Autodesk Inventor part; units mm, degrees
ref_plane "YZ Plane" through (0, 0, 0) normal (1, 0, 0) x (0, 1, 0)
ref_plane "XZ Plane" through (0, 0, 0) normal (0, 1, 0) x (-1, 0, 0)
ref_plane "XY Plane" through (0, 0, 0) normal (0, 0, 1) x (1, 0, 0)
sketch "Эскиз1" plane through (0, 0, 0) normal (0, 0, 1) x (1, 0, 0)
  line L0 (0, 0) -> (10.2, 0)
  line L1 (10.2, 0) -> (10.2, -6.1)
  line L2 (10.2, -6.1) -> (0, -6.1)
  line L3 (0, -6.1) -> (0, 0)
  line L4 (10.2, -6.1) -> (2.2, -6.1)
  line L5 (2.2, -6.1) -> (2.2, -7.1)
  line L6 (2.2, -7.1) -> (10.2, -7.1)
  line L7 (10.2, -7.1) -> (10.2, -6.1)
  dimension "d0" = 10.2
  dimension "d1" = 6.1
  dimension "d2" = 8
  dimension "d3" = 1
extrude "Выдавливание1" add sketch "Эскиз1" along normal blind 0.8
sketch "Эскиз2" plane through (0, 0, 0.8) normal (0, 0, 1) x (1, 0, 0)
  line L0 (2.2, -7.1) -> (10.2, -7.1)
  line L1 (10.2, -7.1) -> (10.2, -3.9)
  line L2 (10.2, -7.1) -> (10.2, 0)
  line L3 (10.2, -3.9) -> (5.1, -3.9)
  line L4 (0, 0) -> (0, -6.1)
  circle A0 centre (5.1, -3.9) radius 1.9
  dimension "d6" = 3.2
  dimension "d7" = 5.1
  dimension "d8" = 3.8
extrude "Выдавливание2" cut sketch "Эскиз2" against normal blind 0.8
properties part number "shayba kvadrat"
Could you check a few things on this model? Use its own coordinates, in mm. Round coordinates to 2 decimals unless told otherwise and drop trailing zeros. Order: outer loops, then holes, each group sorted by start corner. A loop starts at its lowest first (then second) coordinate and runs counter-clockwise, first axis right, second up. Notation, with made-up numbers: M 73.5,76.5 L 78.5,76.5 A17 ccw 78.5,103.5 Z; hole C 32,30.5 d3. An arc over 180 degrees is marked long. One line per item, written item: value.
(1) Imagine slicing it at A-A (y = -3.9). Write out the boundary of the cut face in (x, z).
Ans:
outline: M 0,0 L 3.2,0 L 3.2,0.8 L 0,0.8 Z; M 7,0 L 10.2,0 L 10.2,0.8 L 7,0.8 Z
(2) Imagine slicing it at D-D (x = 2). Write out the boundary of the cut face in (y, z), and give its area (3 significant figures).
Ans:
outline: M -6.1,0 L 0,0 L 0,0.8 L -6.1,0.8 Z
area: 4.88 mm^2
(3) I need wall thicknesses on line 1 along Y through (x, z) = (5.1, 0.6); line 2 along X through (y, z) = (-5.5, 0.3); line 3 along Y through (x, z) = (1, 0.4). Which ranges of each line are inside material? Lowest first, please. Write a range as from..to.
Ans:
line 1: y = -7.1..-5.8, -2..0
line 2: x = 0..4.08, 6.12..10.2
line 3: y = -6.1..0
(4) Imagine slicing it at C-C (z = 0.4). Write out the boundary of the cut face in (x, y), and give its area (3 significant figures).
Ans:
outline: M 0,-6.1 L 2.2,-6.1 L 2.2,-7.1 L 10.2,-7.1 L 10.2,0 L 0,0 Z; hole C 5.1,-3.9 d3.8
area: 58.9 mm^2
(5) Imagine slicing it at B-B (x = 5.1). Write out the boundary of the cut face in (y, z), and give its area (3 significant figures).
Ans:
outline: M -7.1,0 L -5.8,0 L -5.8,0.8 L -7.1,0.8 Z; M -2,0 L 0,0 L 0,0.8 L -2,0.8 Z
area: 2.64 mm^2
